from build123d import *

# Parameters (mm, degrees)
SKETCH1_R           = 2.125
BOSS_EXTRUDE1_DEPTH = 3.175
SKETCH4_W           = 34
SKETCH4_H           = 38.35
BOSS_EXTRUDE2_DEPTH = 3.175
BOSS_EXTRUDE3_REACH = 57.962
SKETCH6_W           = 34
SKETCH6_H           = 7.4
BOSS_EXTRUDE4_DEPTH = 11.7
FILLET1_START       = -36
FILLET1_DEPTH       = 40
FILLET1_START_2     = -35.175
FILLET1_2_DEPTH     = 3.175
FILLET1_3_DEPTH     = 3.175
FILLET1_START_3     = -32.3353435
FILLET1_4_DEPTH     = 32.635
SKETCH7_W           = 34
SKETCH7_H           = 20.3
CUT_EXTRUDE1_DEPTH  = 0.3
SKETCH8_R           = 1.7
CUT_EXTRUDE2_DEPTH  = 60.108893155


with BuildPart() as part:
    # Sketch1 → Boss-Extrude1 (new body)
    with BuildSketch(Plane.XY):
        Polygon((0, 0), (-18, 0), (-18, -6), (-34, -6), (-34, 0), (-34, 24), (0, 24), align=None)
        with Locations((-8, 4)):
            Circle(SKETCH1_R, mode=Mode.SUBTRACT)
    boss_extrude1 = extrude(amount=BOSS_EXTRUDE1_DEPTH)

    # Sketch4 → Boss-Extrude2 (add)
    with BuildSketch(Plane(origin=(0, 24, 0), x_dir=(1, 0, 0), z_dir=(0, 1, 0))):
        with Locations((-17, 16)):
            Rectangle(SKETCH4_W, SKETCH4_H)
    extrude(amount=BOSS_EXTRUDE2_DEPTH)

    # Mirror2: Boss-Extrude1 across plane
    add(boss_extrude1.mirror(Plane(origin=(0, 0, -16), x_dir=(1, 0, 0), z_dir=(0, 0, -1))))

    # Sketch5 → Boss-Extrude3 (add, up to next)
    with BuildSketch(Plane(origin=(0, 0, 0), x_dir=(-1, 0, 0), z_dir=(0, 0, -1)), mode=Mode.PRIVATE) as boss_extrude3_sk1:
        with BuildLine():
            Line((18, 9), (18, 16.6))
            Line((18, 16.6), (34, 16.6))
            Line((34, 16.6), (34, -6))
            Line((34, -6), (18, -6))
            Line((18, -6), (18, -1))
            ThreePointArc((18, -1), (19.755002002, 4), (18, 9))
        make_face()
    boss_extrude3_tool1 = extrude(boss_extrude3_sk1.sketch, amount=BOSS_EXTRUDE3_REACH, mode=Mode.PRIVATE) - part.part
    add(boss_extrude3_tool1.solids().sort_by_distance((-26.249904, 5.344559, 0))[0])

    # Sketch6 → Boss-Extrude4 (add)
    with BuildSketch(Plane.XY.offset(-32)):
        with Locations((-17, 20.3)):
            Rectangle(SKETCH6_W, SKETCH6_H)
    extrude(amount=BOSS_EXTRUDE4_DEPTH)

    # Fillet1: read off the stored shape, not the designer's step
    # Fillet1 outline → Fillet1 (cut)
    with BuildSketch(Plane.XY.offset(FILLET1_START)):
        with BuildLine():
            Line((-34, -6), (-32, -6))
            ThreePointArc((-32, -6), (-33.414213562, -5.414213562), (-34, -4))
            Line((-34, -4), (-34, -6))
        make_face()
        with BuildLine():
            Line((-18, -6), (-18, -4))
            ThreePointArc((-18, -4), (-18.585786438, -5.414213562), (-20, -6))
            Line((-20, -6), (-18, -6))
        make_face()
        with BuildLine():
            ThreePointArc((0, 2), (-0.585786438, 0.585786438), (-2, 0))
            Line((-2, 0), (0, 0))
            Line((0, 0), (0, 2))
        make_face()
    extrude(amount=FILLET1_DEPTH, mode=Mode.SUBTRACT)

    # Fillet1 2 outline → Fillet1 2 (add)
    with BuildSketch(Plane.XY.offset(FILLET1_START_2)):
        with BuildLine():
            Line((-16, 0), (-18, 0))
            Line((-18, 0), (-18, -2))
            ThreePointArc((-18, -2), (-17.414213562, -0.585786438), (-16, 0))
        make_face()
    extrude(amount=FILLET1_2_DEPTH)

    # Fillet1 3 outline → Fillet1 3 (add)
    with BuildSketch(Plane.XY):
        with BuildLine():
            Line((-16, 0), (-18, 0))
            Line((-18, 0), (-18, -2))
            ThreePointArc((-18, -2), (-17.414213562, -0.585786438), (-16, 0))
        make_face()
    extrude(amount=FILLET1_3_DEPTH)

    # Fillet1 4 outline → Fillet1 4 (add)
    with BuildSketch(Plane.XY.offset(FILLET1_START_3)):
        with BuildLine():
            ThreePointArc((-18, -2), (-17.957937252, -1.591978289), (-17.833518283, -1.201119092))
            ThreePointArc((-17.833518283, -1.201119092), (-17.91757965, -1.101238744), (-18, -1))
            Line((-18, -1), (-18, -2))
        make_face()
    extrude(amount=FILLET1_4_DEPTH)

    # Sketch7 → Cut-Extrude1 (cut)
    with BuildSketch(Plane.XZ.offset(-24)):
        with Locations((-17, -10.15)):
            Rectangle(SKETCH7_W, SKETCH7_H)
    extrude(amount=-CUT_EXTRUDE1_DEPTH, mode=Mode.SUBTRACT)

    # Sketch8 → Cut-Extrude2 (cut, through all)
    with BuildSketch(Plane(origin=(0, 27.175, 0), x_dir=(1, 0, 0), z_dir=(0, 1, 0))):
        with Locations(Location((-15, 10, 0), (0, 0, 180))):
            Circle(SKETCH8_R)
        with Locations(Location((-27, 10, 0), (0, 0, 180))):
            Circle(SKETCH8_R)
        with Locations(Location((-6, 10, 0), (0, 0, 180))):
            Circle(SKETCH8_R)
    extrude(amount=-CUT_EXTRUDE2_DEPTH, mode=Mode.SUBTRACT)


solid = part.part
The listing builds one solid part. Answer for the finished solid, in the listing's coordinates (mm). A direction names the side the tool comes from. Give positions to 0.01 mm unless a question says otherwise; leave off trailing zeros. Write each loop counter-clockwise with the first axis right and the second up, starting at its lowest first coordinate (ties: lowest second). Pieces come first, ordered by that corner, then holes.
Item 1: Section C-C, the plane x = -27 is taken. Write down the section's boundary in (y, z) (3 decimals), plus the area to 3 significant figures.
Item 2: Section B-B, the plane x = -31.5 is taken. Write down the section's boundary in (y, z) (3 decimals).
Item 3: Flat-ended cylindrical pins translate along their axes: P1, Ø6, axis at x = -10, z = -15, coming from the -Y side; P2, Ø1.6, axis at y = -2.5, z = -8, coming from the +X side; P3, Ø13, axis at x = -7.5, z = -28.5, coming from the -Y side. Find the tip coordinate at first contact, or state that the pin passes through.
Item 4: Determine the mould class of faces 1 (the cylindrical face through (-16.57, 25.76, -10.65)), 2 (the flat face through (-24, 16.6, -10)), 3 (the cylindrical face through (-17.937, -1.504, -16.268)) for opening direction X: released by +X, released by -X, zero draft, split by the parting line, or undercut.
Item 5: Section D-D, the plane z = -14.5 is taken. Write down the section's boundary in (x, y) (3 decimals).
Item 6: Find the intervals of material crossed by line 1 along Z through (x, y) = (-9, 20.5) (3 decimals); line 2 along Z through (x, y) = (-15.5, 12.5) (3 decimals); line 3 along Y through (x, z) = (-11.5, -28) (3 decimals), in increasing order.
Item 7: Which of the six approach directions +Z, -Z, +X, -X, +Y, -Y give full straight-line access (tool end or side, diameter ignored) to faces 4 (the cylindrical face through (-28.57, 5.46, -10.65)), 5 (the flat face through (-18, -3, -16)), 6 (the flat face through (-17, 24.3, -10)), 7 (the flat face through (-18, 13, -16)), 8 (the cylindrical face through (-7.019, 2.115, 1.565))?
Item 8: Section A-A, the plane y = 21.5 is taken. Write down the section's boundary in (x, z) (3 decimals), plus the area to 3 significant figures.
Completed:
1. outline: (-6, -35.175) - (27.175, -35.175) - (27.175, -11.7) - (24.3, -11.7) - (24.3, -20.3) - (16.6, -20.3) - (16.6, -11.7) - (-6, -11.7) - close; (-6, -8.3) - (16.6, -8.3) - (16.6, 0) - (24.3, 0) - (24.3, -8.3) - (27.175, -8.3) - (27.175, 3.175) - (-6, 3.175) - close
1. area: 1,030 mm2
2. outline: (-6, -35.175) - (27.175, -35.175) - (27.175, 3.175) - (-6, 3.175) - close; hole (16.6, -20.3) - (24.3, -20.3) - (24.3, 0) - (16.6, 0) - close
3. P1: stops at y = 24.3
3. P2: stops at x = -17.98
3. P3: stops at y = 0
4. face 1: undercut
4. face 2: zero draft
4. face 3: released by +X
5. outline: (-34, -4) arc R2 ccw to (-32, -6) - (-20, -6) arc R2 ccw to (-18, -4) - (-18, -2) arc R2 cw to (-17.834, -1.201) arc R8 cw to (-18, 9) - (-18, 16.6) - (-34, 16.6) - close; (-34, 24.3) - (0, 24.3) - (0, 27.175) - (-34, 27.175) - close
6. line 1: z = -35.175 to -20.3, 0 to 3.175
6. line 2: z = -35.175 to -32, 0 to 3.175
6. line 3: y = 16.6 to 27.175
7. face 4: +Y, -Y
7. face 5: +Z, -Z, +X, -Y
7. face 6: +X, -X
7. face 7: +X
7. face 8: +Z, -Z
8. outline: (-34, -35.175) - (0, -35.175) - (0, -20.3) - (-34, -20.3) - close; (-34, 0) - (0, 0) - (0, 3.175) - (-34, 3.175) - close
8. area: 614 mm2
